CAD build for the part. Positions are in the model's coordinates, mm. Face numbers are marked on the shaded views. A direction names the side the tool comes from. Give positions to 0.01 mm unless a question says otherwise; leave off trailing zeros. Write each loop counter-clockwise with the first axis right and the second up, starting at its lowest first coordinate (ties: lowest second). Pieces come first, ordered by that corner, then holes. Notation, with made-up numbers: M -32.5,46 L 13.5,46 A31 ccw 13.5,71 Z; hole C -29.5,-38.5 d1. An arc over 180 degrees is marked long. One line per question, with ' | ' between items. Start each with the question number.
1. Cut at D-D, the plane x = -24. Write the cut outline in (y, z).
2. Which spindle directions (+Z, -Z, +X, -X, +Y, -Y) get a long thin tool onto all of the face, cutting with end or side? Do the marked faces 1, 2 and 3. Say none if no direction does.
3. Wall check: L1, parallel to X at y = 2.5, z = 11.5; L2, parallel to Y at x = -33.7, z = 0; L3, parallel to X at y = 14, z = 19.5. Give the ranges that are in metal, low to high.
4. Pull direction Y, two halves, no side cores. Call the marked faces 4, 5, 6 and 7: released by +Y, released by -Y, zero draft, split by the parting line, or undercut.
5. Cut at A-A, the plane z = 22.5. Write the cut outline in (x, y).
6. Cut at B-B, the plane x = -45.5. Count the separate pieces of the cut face and the enclosed holes in it, then the cut area to 3 significant figures.
7. Flat gauge pins, fed straight in: pin 1 (7 mm diameter, centred on y = 17.06, z = -17.06, fed in from +X); pin 2 (13.5 mm diameter, centred on x = -14.605, z = 0, fed in from +Y); pin 3 (1.5 mm diameter, centred on x = -38.5, z = 9, fed in from -Y); pin 4 (16.5 mm diameter, centred on y = 1, z = 1, fed in from -X). Where does each tip first touch, or does it go through?
8. Cut at C-C, the plane y = -24.13. Write the cut outline in (x, z), then the cut area to 3 significant figures.
```python
from build123d import *

# Parameters (mm, degrees)
SKETCH2_R                = 20.32
BOSS_EXTRUDE1_DEPTH      = 49.53
SKETCH3_R                = 29.21
SKETCH3_R_2              = 19.05
BOSS_EXTRUDE2_DEPTH      = 5.08
M5_CLEARANCE_HOLE1_D     = 5.5
M5_CLEARANCE_HOLE1_DEPTH = 5.08
SKETCH6_W                = 11.43
SKETCH6_H                = 25.4
CUT_EXTRUDE1_DEPTH       = 1.27
SKETCH9_R                = 16.7132
SKETCH9_R_2              = 14.1478
CUT_EXTRUDE2_DEPTH       = 1.27


# Read off the part's stored shape, not the designer's step: 1/8 NPT Tapped Hole1
with BuildPart() as part:
    # Sketch2 → Boss-Extrude1 (new body)
    with BuildSketch(Plane(origin=(0, 0, 0), x_dir=(0, 0, -1), z_dir=(1, 0, 0))):
        Circle(SKETCH2_R)
    extrude(amount=-BOSS_EXTRUDE1_DEPTH)

    # Sketch1 → Cut-Revolve1 (revolve, cut)
    with BuildSketch(Plane.XY):
        Polygon((-30.6578, 10.6299), (-30.6578, 11.9507), (-33.02, 11.9507), (-33.02, 10.6299), (-34.29, 10.6299), (-34.29, 12.7), (-49.53, 12.7), (-49.53, 0), (0, 0), (0, 12.7), (-6.35, 12.7), (-6.35, 10.6299), (-26.5176, 10.6299), (-26.5176, 11.9507), (-28.8798, 11.9507), (-28.8798, 10.6299), align=None)
    revolve(axis=Axis((0, 0, 0), (-1, 0, 0)), mode=Mode.SUBTRACT)

    # Sketch3 → Boss-Extrude2 (add)
    with BuildSketch(Plane.ZY.offset(49.53)):
        Circle(SKETCH3_R)
        Circle(SKETCH3_R_2, mode=Mode.SUBTRACT)
    extrude(amount=-BOSS_EXTRUDE2_DEPTH)

    # M5 Clearance Hole1
    with Locations(Plane(origin=(-44.45, 0, 0), x_dir=(0, 0, -1), z_dir=(1, 0, 0))):
        with Locations((0, 24.13), (0, 0), (17.06248663, 17.06248663), (24.13, 0), (17.06248663, -17.06248663), (0, -24.13), (-17.06248663, -17.06248663), (-24.13, 0), (-17.06248663, 17.06248663)):
            Hole(M5_CLEARANCE_HOLE1_D / 2, depth=M5_CLEARANCE_HOLE1_DEPTH)

    # Sketch6 → Cut-Extrude1 (cut)
    with BuildSketch(Plane(origin=(0, 20.32, 0), x_dir=(1, 0, 0), z_dir=(0, 1, 0))):
        with Locations((-14.605, 0)):
            Rectangle(SKETCH6_W, SKETCH6_H)
    extrude(amount=-CUT_EXTRUDE1_DEPTH, mode=Mode.SUBTRACT)

    # 1/8 NPT Tapped Hole1 outline → 1/8 NPT Tapped Hole1 (revolve, cut)
    with BuildSketch(Plane(origin=(-14.605, 0, 0), x_dir=(1, 0, 0), z_dir=(0, 0, 1))):
        Polygon((0, 9.757655132), (4.2164, 9.757655132), (4.2164, 12.192), (4.537401096, 12.192), (4.7427388, 19.05), (0, 19.05), align=None)
    revolve(axis=Axis((-14.605, 0, 0), (0, 1, 0)), mode=Mode.SUBTRACT)

    # Sketch9 → Cut-Extrude2 (cut)
    with BuildSketch(Plane.ZY.offset(49.53)):
        Circle(SKETCH9_R)
        Circle(SKETCH9_R_2, mode=Mode.SUBTRACT)
    extrude(amount=-CUT_EXTRUDE2_DEPTH, mode=Mode.SUBTRACT)


solid = part.part
```
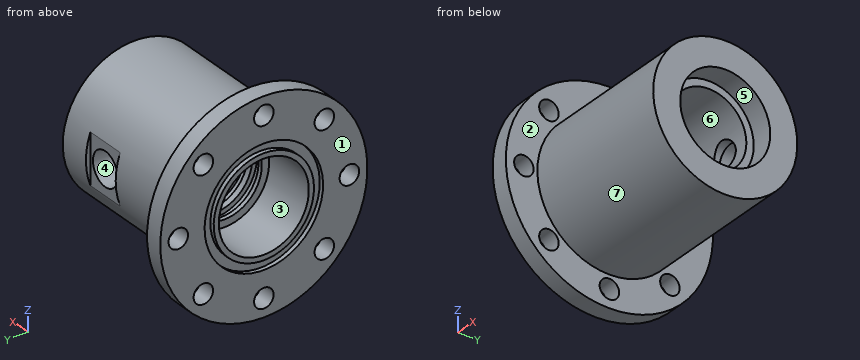
Here are the results:
1) outline: C 0,0 d40.64; hole C 0,0 d21.26
2) face 1: +Z, -Z, -X, +Y, -Y | face 2: +X | face 3: -X
3) L1: -34.29 to -33.02, -30.66 to -28.88, -26.52 to -6.35 | L2: -20.32 to -10.63, 10.63 to 20.32 | L3: -49.53 to -44.45
4) face 4: released by +Y | face 5: undercut | face 6: undercut | face 7: split by the parting line
5) outline: M -49.53,-18.63 L -44.45,-18.63 L -44.45,-2.21 L -49.53,-2.21 Z; M -49.53,2.21 L -44.45,2.21 L -44.45,18.63 L -49.53,18.63 Z
6) separate pieces: 1 | enclosed holes: 9 | area: 1,980 mm^2
7) pin 1: x = -44.45 | pin 2: y = 20.32 | pin 3: y = -18.57 | pin 4: through
8) outline: M -49.53,-16.46 L -44.45,-16.46 L -44.45,-2.75 L -49.53,-2.75 Z; M -49.53,2.75 L -44.45,2.75 L -44.45,16.46 L -49.53,16.46 Z | area: 139 mm^2
